Source: three-view drawing plus pictorial views. Frame: mm from the lowest corner of the part. Give positions to 0.01 mm unless a question says otherwise; leave off trailing zeros. Loops run counter-clockwise (first coordinate to the right, second up) from the corner with the lowest first, then second, coordinate; pieces in that order, holes last. Notation, with made-up numbers: (45, -15) - (75, -15) arc R12 cw to (75, 6) - close; hole circle Ø4 at (-2, 74.5). An arc over 180 degrees is marked (long way). Answer in a Markdown table with one row per item.
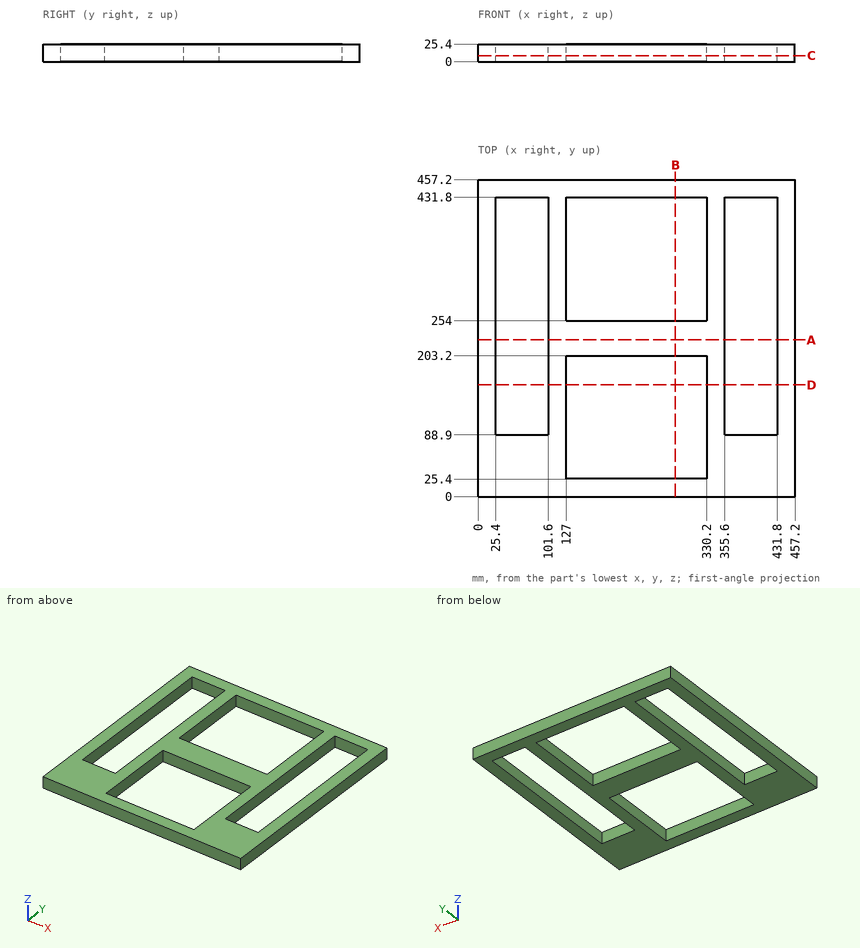
Q1. Cut plane C-C (z = 8.5). Output: boundary loops of the cut face in (x, y).
Check values:
| item | result |
|---|---|
| outline | (0, 0) - (457.2, 0) - (457.2, 457.2) - (0, 457.2) - close; hole (25.4, 88.9) - (101.6, 88.9) - (101.6, 431.8) - (25.4, 431.8) - close; hole (127, 25.4) - (330.2, 25.4) - (330.2, 203.2) - (127, 203.2) - close; hole (127, 254) - (330.2, 254) - (330.2, 431.8) - (127, 431.8) - close; hole (355.6, 88.9) - (431.8, 88.9) - (431.8, 431.8) - (355.6, 431.8) - close |
Q2. Cut plane B-B (x = 284.5). Output: boundary loops of the cut face in (y, z).
Check values:
| item | result |
|---|---|
| outline | (0, 0) - (25.4, 0) - (25.4, 25.4) - (0, 25.4) - close; (203.2, 0) - (254, 0) - (254, 25.4) - (203.2, 25.4) - close; (431.8, 0) - (457.2, 0) - (457.2, 25.4) - (431.8, 25.4) - close |
Q3. Cut plane D-D (y = 161). Output: boundary loops of the cut face in (x, z), and give its area (3 significant figures).
Check values:
| item | result |
|---|---|
| outline | (0, 0) - (25.4, 0) - (25.4, 25.4) - (0, 25.4) - close; (101.6, 0) - (127, 0) - (127, 25.4) - (101.6, 25.4) - close; (330.2, 0) - (355.6, 0) - (355.6, 25.4) - (330.2, 25.4) - close; (431.8, 0) - (457.2, 0) - (457.2, 25.4) - (431.8, 25.4) - close |
| area | 2,580 mm² |
Q4. Material intervals for line 1 along X through (y, z) = (124.5, 13); line 2 along Y through (x, z) = (276, 3.25); line 3 along X through (y, z) = (253, 16.5), sorted ascending.
Check values:
| item | result |
|---|---|
| line 1 | 0 to 25.4, 101.6 to 127, 330.2 to 355.6, 431.8 to 457.2 |
| line 2 | 0 to 25.4, 203.2 to 254, 431.8 to 457.2 |
| line 3 | 0 to 25.4, 101.6 to 355.6, 431.8 to 457.2 |
Q5. Cut plane A-A (y = 226). Output: boundary loops of the cut face in (x, z).
Check values:
| item | result |
|---|---|
| outline | (0, 0) - (25.4, 0) - (25.4, 25.4) - (0, 25.4) - close; (101.6, 0) - (355.6, 0) - (355.6, 25.4) - (101.6, 25.4) - close; (431.8, 0) - (457.2, 0) - (457.2, 25.4) - (431.8, 25.4) - close |
